Drawing for the job (mm, zero at the part's lowest x, y, z). Round coordinates to 2 decimals unless told otherwise and drop trailing zeros. Write each loop counter-clockwise with the first axis right and the second up, starting at its lowest first coordinate (ties: lowest second). Pieces come first, ordered by that corner, then holes. Notation, with made-up numbers: (-1.75, 13.5) - (50.25, 13.5) arc R19 cw to (50.25, 18.5) - close; hole circle Ø6 at (87, 59). An arc over 180 degrees is marked (long way). Answer in a Markdown table with one row per item.
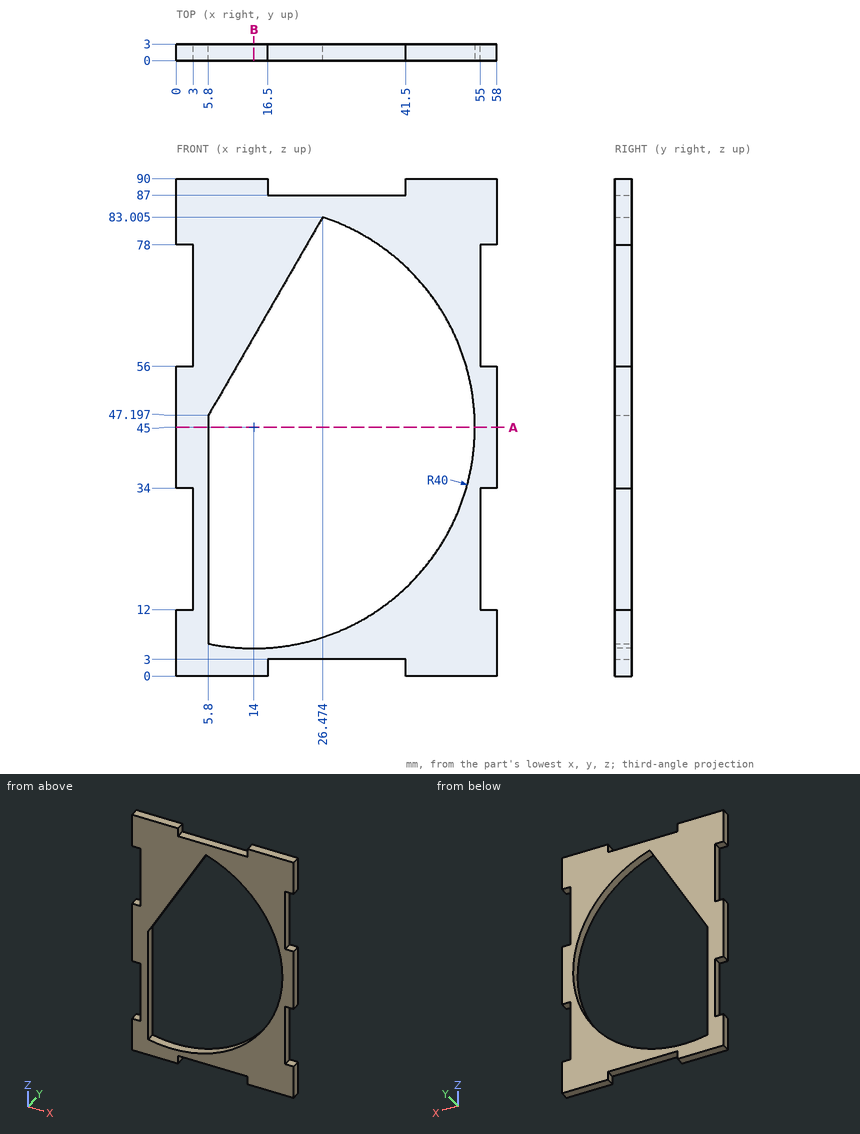
Q1. Saw through at A-A on z = 45. List the corners of the cut face in (x, y).
Computed:
| item | result |
|---|---|
| outline | (0, 0) - (5.8, 0) - (5.8, 3) - (0, 3) - close; (54, 0) - (58, 0) - (58, 3) - (54, 3) - close |
Q2. Drill centre lines: line 1 (Z direction, x = 42, y = 1.3) (1 decimal); line 2 (X direction, y = 1.7, z = 25); line 3 (Z direction, x = 50, y = 2.25) (1 decimal). Where is each one in solid material? Low to high.
Computed:
| item | result |
|---|---|
| line 1 | z = 0 to 16.4, 73.6 to 90 |
| line 2 | x = 3 to 5.8, 48.64 to 55 |
| line 3 | z = 0 to 27.6, 62.4 to 90 |
Q3. Saw through at B-B on x = 14. List the corners of the cut face in (y, z).
Computed:
| item | result |
|---|---|
| outline | (0, 0) - (3, 0) - (3, 5) - (0, 5) - close; (0, 61.4) - (3, 61.4) - (3, 90) - (0, 90) - close |
Q4. Flat gauge pins, fed straight in: pin 1 (0.9 mm diameter, centred on y = 2, z = 72.5, fed in from +X); pin 2 (0.9 mm diameter, centred on y = 1.5, z = 26.5, fed in from -X); pin 3 (1.5 mm diameter, centred on x = 33.5, y = 1.5, fed in from -Z). Where does each tip first touch, or does it go through?
Computed:
| item | result |
|---|---|
| pin 1 | stops at x = 55 |
| pin 2 | stops at x = 3 |
| pin 3 | stops at z = 3 |
